from build123d import *

# Parameters (mm, degrees)
SKETCH1_W           = 50
SKETCH1_H           = 22.5
BOSS_EXTRUDE1_DEPTH = 35
SKETCH2_R           = 4.5
CUT_EXTRUDE1_DEPTH  = 35
CUT_EXTRUDE2_DEPTH  = 5.5
SKETCH4_W           = 10
SKETCH4_H           = 5
SKETCH4_W_2         = 10.024005515
SKETCH4_H_2         = 4
BOSS_EXTRUDE2_DEPTH = 12.2
SKETCH5_W           = 7.3
SKETCH5_H           = 22.5
CUT_EXTRUDE3_DEPTH  = 49.98879974


with BuildPart() as part:
    # Sketch1 → Boss-Extrude1 (new body)
    with BuildSketch(Plane.XY):
        Rectangle(SKETCH1_W, SKETCH1_H)
    extrude(amount=BOSS_EXTRUDE1_DEPTH)

    # Sketch2 → Cut-Extrude1 (cut)
    with BuildSketch(Plane.XY.offset(35)):
        with Locations((10, -5)):
            Circle(SKETCH2_R)
        with Locations(Location((-10, -5, 0), (0, 0, 180))):
            Circle(SKETCH2_R)
    extrude(amount=-CUT_EXTRUDE1_DEPTH, mode=Mode.SUBTRACT)

    # Sketch3 → Cut-Extrude2 (cut)
    with BuildSketch(Plane(origin=(0, 11.25, 0), x_dir=(1, 0, 0), z_dir=(0, 1, 0))):
        with BuildLine():
            Line((25, -19.75), (13.311179512, -19.75))
            ThreePointArc((13.311179512, -19.75), (0, -31), (-13.311179512, -19.75))
            Line((-13.311179512, -19.75), (-25, -19.75))
            Line((-25, -19.75), (-25, -15.25))
            Line((-25, -15.25), (-13.311179512, -15.25))
            ThreePointArc((-13.311179512, -15.25), (0, -4), (13.311179512, -15.25))
            Line((13.311179512, -15.25), (25, -15.25))
            Line((25, -15.25), (25, -19.75))
        make_face()
    extrude(amount=-CUT_EXTRUDE2_DEPTH, mode=Mode.SUBTRACT)

    # Sketch4 → Boss-Extrude2 (add)
    with BuildSketch(Plane(origin=(0, 11.25, 0), x_dir=(1, 0, 0), z_dir=(0, 1, 0))):
        with Locations((20, -2.5)):
            Rectangle(SKETCH4_W, SKETCH4_H)
        with Locations((19.987997243, -8.75)):
            Rectangle(SKETCH4_W_2, SKETCH4_H_2)
        with Locations((19.987997243, -26.25)):
            Rectangle(SKETCH4_W_2, SKETCH4_H_2)
        with Locations((20, -32.5)):
            Rectangle(SKETCH4_W, SKETCH4_H)
    extrude(amount=BOSS_EXTRUDE2_DEPTH)

    # Sketch5 → Cut-Extrude3 (cut, through all)
    with BuildSketch(Plane(origin=(0, 0, 0), x_dir=(-1, 0, 0), z_dir=(0, 0, -1))):
        with Locations((21.35, 0)):
            Rectangle(SKETCH5_W, SKETCH5_H)
    extrude(amount=-CUT_EXTRUDE3_DEPTH, mode=Mode.SUBTRACT)


solid = part.part
Input: part model. Units: mm. Frame: model coordinates. A direction names the side the tool comes from. Round coordinates to 2 decimals unless told otherwise and drop trailing zeros. Write each loop counter-clockwise with the first axis right and the second up, starting at its lowest first coordinate (ties: lowest second). Pieces come first, ordered by that corner, then holes.
1) Cut plane A-A (y = 18). Return the cut outline in (x, z).
2) Reachability of faces 1 (the flat face through (20, 17, 6.75)), 2 (the flat face through (-1, 5.75, 17)), 3 (the flat face through (8, 2, 35)) from +Z, -Z, +X, -X, +Y, -Y: full face, straight path, thin tool, end or side. Return the list, or none.
3) Contact query for flat-ended pins moving along their axis: P1, Ø1.5, axis at x = -2.5, y = 5, coming from the -Z side; P2, Ø2, axis at y = 18, z = 9, coming from the -X side; P3, Ø17, axis at x = 4.5, z = 27, coming from the +Y side; P4, Ø3, axis at x = -9, z = 14.5, coming from the +Y side. Output: stop coordinate, or through.
4) Draft query along Y for faces 4 (the flat face through (19, 9, 15.25)), 5 (the cylindrical face through (-14.16, -3.28, 17.74)), 6 (the flat face through (3, -11.25, 17)). Return one class per face: pulls with the +Y half, pulls with the -Y half, needs draft (parallel to the pull), parting line crosses it, or undercut.
5) Cut plane C-C (x = -8.5). Return the cut outline in (y, z).
6) Cut plane B-B (y = -5). Return the cut outline in (x, z), then the cut area to 4 significant figures.
7) Cut plane D-D (z = 25). Return the cut outline in (x, y), then the cut area to 3 significant figures.
8) Ray query, L1, parallel to Y at x = -10, z = 28.5; L2, parallel to Y at x = 10, z = 10; L3, parallel to X at y = -7, z = 22. Return the intervals inside material, ascending.
Geometry says:
1. outline: (14.98, 6.75) - (25, 6.75) - (25, 10.75) - (14.98, 10.75) - close; (14.98, 24.25) - (25, 24.25) - (25, 28.25) - (14.98, 28.25) - close; (15, 0) - (25, 0) - (25, 5) - (15, 5) - close; (15, 30) - (25, 30) - (25, 35) - (15, 35) - close
2. face 1: +X, -X, +Y
2. face 2: +Y
2. face 3: +Z, +X, -X, +Y, -Y
3. P1: stops at z = 0
3. P2: stops at x = 14.98
3. P3: stops at y = 11.25
3. P4: stops at y = 5.75
4. face 4: needs draft
4. face 5: undercut
4. face 6: pulls with the -Y half
5. outline: (-11.25, 0) - (-9.24, 0) - (-9.24, 35) - (-11.25, 35) - close; (-0.76, 0) - (11.25, 0) - (11.25, 7.01) - (5.75, 7.01) - (5.75, 27.99) - (11.25, 27.99) - (11.25, 35) - (-0.76, 35) - close
6. outline: (-17.7, 0) - (-14.5, 0) - (-14.5, 35) - (-17.7, 35) - close; (-5.5, 0) - (5.5, 0) - (5.5, 35) - (-5.5, 35) - close; (14.5, 0) - (25, 0) - (25, 35) - (14.5, 35) - close
6. area: 864.5 mm2
7. outline: (-17.7, -11.25) - (25, -11.25) - (25, 23.45) - (14.98, 23.45) - (14.98, 11.25) - (11.22, 11.25) - (11.22, 5.75) - (-11.22, 5.75) - (-11.22, 11.25) - (-17.7, 11.25) - close; hole circle Ø9 at (-10, -5); hole circle Ø9 at (10, -5)
7. area: 832 mm2
8. L1: y = -11.25 to -9.5, -0.5 to 11.25
8. L2: y = -11.25 to -9.5, -0.5 to 5.75
8. L3: x = -17.7 to -14.03, -5.97 to 5.97, 14.03 to 25
